```python
from build123d import *

# Parameters (mm, degrees)
F0_W     = 120
F0_H     = 60
F1_DEPTH = 25
F2_W     = 60
F2_H     = 60
F3_DEPTH = 10
F4_W     = 15
F4_H     = 60
F5_DEPTH = 10
F6_W     = 15
F6_H     = 15
F7_DEPTH = 20
F9_DEPTH = 25.001


with BuildPart() as f1:
    # F0 (on Top) → F1 (new body)
    with BuildSketch(Plane.XY):
        Rectangle(F0_W, F0_H)
    extrude(amount=F1_DEPTH)

    # F2 (on face) → F3 (cut)
    with BuildSketch(Plane(origin=(0, 0, 0), x_dir=(1, 0, 0), z_dir=(0, 0, -1))):
        with Locations((30, 0)):
            Rectangle(F2_W, F2_H)
    extrude(amount=-F3_DEPTH, mode=Mode.SUBTRACT)

    # F4 (on face) → F5 (join)
    with BuildSketch(Plane.XY.offset(25)):
        with Locations((-52.5, 0)):
            Rectangle(F4_W, F4_H)
    extrude(amount=F5_DEPTH)

    # F6 (on face) → F7 (join)
    with BuildSketch(Plane.XY.offset(25)):
        with Locations((52.5, -22.5)):
            Rectangle(F6_W, F6_H)
        with Locations((52.5, 22.5)):
            Rectangle(F6_W, F6_H)
    extrude(amount=F7_DEPTH)

    # F8 (on face) → F9 (cut, through all)
    with BuildSketch(Plane.XY.offset(25)):
        with BuildLine():
            Line((-25, 10), (-25, -10))
            ThreePointArc((-25, -10), (-17.9289321881, -7.0710678119), (-15, 0))
            ThreePointArc((-15, 0), (-17.9289321881, 7.0710678119), (-25, 10))
        make_face()
        with BuildLine():
            ThreePointArc((-25, 10), (-35, 0), (-25, -10))
            Line((-25, -10), (-25, 10))
        make_face()
        with BuildLine():
            ThreePointArc((20, 10), (10, 0), (20, -10))
            Line((20, -10), (20, 10))
        make_face()
        with BuildLine():
            Line((20, 10), (20, -10))
            ThreePointArc((20, -10), (27.0710678119, -7.0710678119), (30, 0))
            ThreePointArc((30, 0), (27.0710678119, 7.0710678119), (20, 10))
        make_face()
    extrude(amount=-F9_DEPTH, mode=Mode.SUBTRACT)


solid = f1.part
```
For this review, take the finished solid that the model builds, in its own axes (mm). A direction names the side the tool comes from. Round coordinates to 2 decimals unless told otherwise and drop trailing zeros. Loops run counter-clockwise (first coordinate to the right, second up) from the corner with the lowest first, then second, coordinate; pieces in that order, holes last.
(1) We need section D-D (y = -22.5). Give the boundary of the cut face in (x, z), plus the area to 3 significant figures.
Returned:
outline: (-60, 0) - (0, 0) - (0, 10) - (60, 10) - (60, 45) - (45, 45) - (45, 25) - (-45, 25) - (-45, 35) - (-60, 35) - close
area: 2,850 mm2
(2) We need section A-A (z = 39). Give the boundary of the cut face in (x, y), plus the area to 3 significant figures.
Returned:
outline: (45, -30) - (60, -30) - (60, -15) - (45, -15) - close; (45, 15) - (60, 15) - (60, 30) - (45, 30) - close
area: 450 mm2
(3) We need section B-B (z = 20.5). Give the boundary of the cut face in (x, y).
Returned:
outline: (-60, -30) - (60, -30) - (60, 30) - (-60, 30) - close; hole circle Ø20 at (-25, 0); hole circle Ø20 at (20, 0)
(4) We need section C-C (x = 27.5). Give the boundary of the cut face in (y, z).
Returned:
outline: (-30, 10) - (-6.61, 10) - (-6.61, 25) - (-30, 25) - close; (6.61, 10) - (30, 10) - (30, 25) - (6.61, 25) - close
(5) Clearance check with flat-ended pins moving along their axes: P1, Ø5, axis at y = -8, z = 31, coming from the +X side; P2, Ø1.5, axis at x = 12, y = -20, coming from the +Z side; P3, Ø16.5, axis at x = -55, y = 4, coming from the +Z side. State where each tip first meets the part, or that it passes through.
Returned:
P1: stops at x = -45
P2: stops at z = 25
P3: stops at z = 35
(6) Mouldability with a two-part tool opening along Y and no side actions: class faces 1 (the flat face through (-1, -30, 17)), 2 (the flat face through (52, 15, 35)), 3 (the flat face through (-1, 30, 17)), 4 (the flat face through (52, 23, 45)) as released by +Y, released by -Y, zero draft, split by the parting line, or undercut.
Returned:
face 1: released by -Y
face 2: undercut
face 3: released by +Y
face 4: zero draft
(7) Wall thickness on line 1 along X through (y, z) = (-9, 12.5); line 2 along Z through (x, y) = (45, -10); line 3 along Z through (x, y) = (46, 22): over which ranges is each line inside the solid? List them lowest first.
Returned:
line 1: x = -60 to -29.36, -20.64 to 15.64, 24.36 to 60
line 2: z = 10 to 25
line 3: z = 10 to 45
(8) Tool access review of faces 5 (the flat face through (36, 0, 10)), 6 (the flat face through (-53, 0, 35)), 7 (the flat face through (52, -15, 35)), 8 (the flat face through (45, 22, 35)): name each direction out of +Z, -Z, +X, -X, +Y, -Y from which nothing blocks a thin tool from reaching the whole face with its end or side.
Returned:
face 5: -Z, +X, +Y, -Y
face 6: +Z, -X, +Y, -Y
face 7: +Z, +X
face 8: +Z, +Y, -Y
